Autodesk Inventor part; units mm, degrees
ref_plane "YZ Plane" through (0, 0, 0) normal (1, 0, 0) x (0, 1, 0)
ref_plane "XZ Plane" through (0, 0, 0) normal (0, 1, 0) x (-1, 0, 0)
ref_plane "XY Plane" through (0, 0, 0) normal (0, 0, 1) x (1, 0, 0)
sketch "Sketch1" plane through (0, 0, 0) normal (0, 0, 1) x (1, 0, 0)
  arc A0 (-44.1071, -48.8952) -> (-20.8929, -67.8977) centre (-32.5, -58.3964) ccw
  arc A1 (-43.869, -48.6061) -> (-44.1071, -48.8952) centre (0, -85) ccw
  line L0 (-36.9673, -34.403) -> (-43.869, -48.6061)
  arc A2 (-36.9673, -34.403) -> (-25, 17.6067) centre (-144, 17.6067) ccw
  line L1 (-25, 17.6067) -> (-25, 75)
  line L2 (-25, 75) -> (25, 75)
  line L3 (25, 75) -> (25, 17.6067)
  arc A3 (25, 17.6067) -> (36.9673, -34.403) centre (144, 17.6067) ccw
  line L4 (43.869, -48.6061) -> (36.9673, -34.403)
  arc A4 (44.1071, -48.8952) -> (43.869, -48.6061) centre (0, -85) ccw
  arc A5 (20.8929, -67.8977) -> (44.1071, -48.8952) centre (32.5, -58.3964) ccw
  arc A6 (20.8929, -67.8977) -> (-20.8929, -67.8977) centre (0, -85) ccw
  circle A7 centre (-16, 24) radius 2.1
  circle A8 centre (16, 60) radius 2.1
  circle A9 centre (-16, 60) radius 2.1
  circle A10 centre (16, 24) radius 2.1
  arc A11 (38.0714, -53.8358) -> (-38.0714, -53.8358) centre (0, -85) ccw
  arc A12 (-38.0714, -53.8358) -> (-26.9286, -62.957) centre (-32.5, -58.3964) ccw
  arc A13 (26.9286, -62.957) -> (-26.9286, -62.957) centre (0, -85) ccw
  arc A14 (26.9286, -62.957) -> (38.0714, -53.8358) centre (32.5, -58.3964) ccw
  circle A15 centre (0, -43) radius 7.1
  line L5 (0, -35.8) -> (0, -50.2) construction
  circle A16 centre (0, -85) radius 21.9
  line L6 (0, -63) -> (0, -213) construction
  line L7 (-42, -63) -> (-42, -213)
  line L8 (42, -213) -> (42, -63)
  arc A17 (42, -63) -> (-42, -63) centre (0, -63) ccw
  arc A18 (-42, -213) -> (42, -213) centre (0, -213) ccw
  point P0 (0, 0)
  point P1 (0, -138)
  dimension "d0" = 14.2
  dimension "d1" = 7.2
  dimension "d2" = 27
  dimension "d3" = 43.8
  dimension "d4" = 42
  dimension "d5" = 150
  dimension "d6" = 20
extrude "Extrusion1" add sketch "Sketch1" against normal blind 8 contours A15 | A16
sketch "Sketch2" plane through (0, -85, 0) normal (0, 0, 1) x (1, 0, 0)
  line L0 (-42, 22) -> (-42, -128)
  arc A0 (42, 22) -> (-42, 22) centre (0, 22) ccw
  line L1 (42, -128) -> (42, 22)
  arc A1 (-42, -128) -> (42, -128) centre (0, -128) ccw
  circle A2 centre (0, 0) radius 21.9
  circle A3 centre (0, 42) radius 7.1
  point P0 (0, 85)
extrude "Extrusion2" add sketch "Sketch2" along normal blind 10 contours A0 L1 A1 L0 | A2 | A3
sketch "Sketch4" plane through (0, -85, 0) normal (0, 0, -1) x (-1, 0, 0)
  circle A0 centre (0, 0) radius 21.9
  circle A1 centre (0, 42) radius 7.1
  arc A2 (-42, -128) -> (42, -128) centre (0, -128) ccw
  line L0 (42, 22) -> (42, -128)
  arc A3 (42, 22) -> (-42, 22) centre (0, 22) ccw
  line L1 (-42, -128) -> (-42, 22)
  arc A4 (-42, -128) -> (42, -128) centre (0, -128) ccw
  line L2 (42, -128) -> (-42, -128)
  line L3 (32, -128) -> (32, 12)
  arc A5 (42, 22) -> (-42, 22) centre (0, 22) ccw
  line L4 (32, 12) -> (42, 22)
  line L5 (0, -128) -> (0, 42) construction
  line L6 (-32, -128) -> (-32, 12)
  line L7 (-32, 12) -> (-42, 22)
  line L8 (22, -128) -> (22, -28)
  line L9 (22, -28) -> (32, -28)
  line L10 (-22, -128) -> (-22, -28)
  line L11 (-22, -28) -> (-32, -28)
  point P0 (0, 85)
  point P1 (-32, -28)
  dimension "d18" = 10
  dimension "d19" = 135
  dimension "d22" = 10
  dimension "d23" = 100
extrude "Extrusion3" cut sketch "Sketch4" against normal blind 10 contours L2 A2 | L1 L7 L6 L2 | L2 L3 L4 L0 | L6 L11 L10 L2 | L2 L8 L9 L3
sketch "Sketch5" plane through (0, -85, 10) normal (0, 0, 1) x (1, 0, 0)
  circle A0 centre (17, -73) radius 2.6
  circle A1 centre (17, -98) radius 2.6
  circle A2 centre (17, -123) radius 2.6
  point P0 (0, 85)
extrude "Extrusion4" cut sketch "Sketch5" against normal through all
ref_plane "Work Plane1" through (0, -85, 5) normal (0, 0, 1) x (1, 0, 0)
mirror "Mirror1" about plane through (0, -85, 5) normal (0, 0, 1) of "Extrusion1"
sketch "Sketch3" plane through (0, -43, -8) normal (0, 0, -1) x (-1, 0, 0)
  circle A0 centre (0, 0) radius 7.1
  point P0 (0, 43)
hole "Hole1" at (0, -43, -8) direction (0, 0, 1) diameter 8.2 end through all
properties part number "17_Khau_noi_tiep_cuoi" material "Stainless Steel, Austenitic"
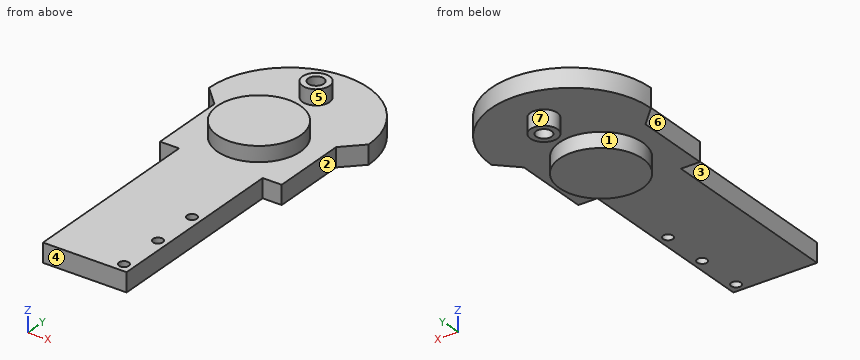
The listing builds one solid part. Answer for the finished solid, in the listing's coordinates (mm). Face numbers are marked on the shaded views. A direction names the side the tool comes from. Coordinates: 2 decimals unless noted, no trailing zeros. Write each loop counter-clockwise with the first axis right and the second up, starting at its lowest first coordinate (ties: lowest second). Pieces come first, ordered by that corner, then holes. Notation, with made-up numbers: M 33,38 L 86,38 A22 ccw 86,47 Z; hole C -35.5,74.25 d8. An arc over 180 degrees is marked long. Use a Markdown table: item, result. Add a question column.
1. Section A-A (x = 0) is taken. Give the vertices of the cut face in (y, z), plus the area to 3 significant figures.
2. Section C-C (y = -183) is taken. Give the vertices of the cut face in (x, z), plus the area to 3 significant figures.
3. Given P1, Ø11, axis at y = -157.5, z = 5.5, coming from the +X side; P2, Ø3, axis at y = -159, z = 6, coming from the -X side; P3, Ø1, axis at y = -79.5, z = 2.5, coming from the +X side, each flat-ended and moving along its own axis, determine where each tip first touches the part or whether it passes through.
4. Straight lines are drawn through the part: line 1 along X through (y, z) = (-158, 2.5); line 2 along Y through (x, z) = (0.5, -7); line 3 along Y through (x, z) = (17, 7.5). For each, find the intervals that lie inside material, in ascending order. Write a range as [from, to].
5. Section D-D (x = 17) is taken. Give the vertices of the cut face in (y, z).
6. For a pull along Y with two mould halves and no side action, classify the marked faces 4, 5, 6 and 7 as +Y half, -Y half, draft (parallel to the pull), parting line (faces both ways), or undercut.
7. Which of the six approach directions +Z, -Z, +X, -X, +Y, -Y give full straight-line access (tool end or side, diameter ignored) to the marked faces 1, 2 and 3?
8. Section B-B (z = -3) is taken. Give the vertices of the cut face in (x, y), plus the area to 3 significant figures.
Data:
| question | item | result |
|---|---|---|
| 1 | outline | M -213,0 L -106.9,0 L -106.9,-8 L -63.1,-8 L -63.1,0 L -50.1,0 L -50.1,-8 L -47.1,-8 L -47.1,18 L -50.1,18 L -50.1,10 L -63.1,10 L -63.1,18 L -106.9,18 L -106.9,10 L -213,10 Z; M -38.9,-8 L -35.9,-8 L -35.9,0 L -21,0 L -21,10 L -35.9,10 L -35.9,18 L -38.9,18 Z |
| 1 | area | 2,630 mm2 |
| 2 | outline | M -22,0 L 14.4,0 L 14.4,10 L -22,10 Z; M 19.6,0 L 22,0 L 22,10 L 19.6,10 Z |
| 2 | area | 388 mm2 |
| 3 | P1 | stops at x = 22 |
| 3 | P2 | stops at x = -22 |
| 3 | P3 | stops at x = 32 |
| 4 | line 1 | x = [-22, 14.4], [19.6, 22] |
| 4 | line 2 | y = [-106.89, -63.11], [-50.08, -47.07], [-38.93, -35.92] |
| 4 | line 3 | y = [-213, -210.6], [-205.4, -185.6], [-180.4, -160.6], [-155.4, -24.59] |
| 5 | outline | M -213,0 L -210.6,0 L -210.6,10 L -213,10 Z; M -205.4,0 L -185.6,0 L -185.6,10 L -205.4,10 Z; M -180.4,0 L -160.6,0 L -160.6,10 L -180.4,10 Z; M -155.4,0 L -98.81,0 L -98.81,-8 L -71.19,-8 L -71.19,0 L -24.59,0 L -24.59,10 L -71.19,10 L -71.19,18 L -98.81,18 L -98.81,10 L -155.4,10 Z |
| 6 | face 4 | -Y half |
| 6 | face 5 | undercut |
| 6 | face 6 | draft |
| 6 | face 7 | undercut |
| 7 | face 1 | -Z |
| 7 | face 2 | +Z, -Z, +X, -Y |
| 7 | face 3 | +Z, -Z, -X, -Y |
| 8 | outline | C 0,-85 d43.8; C 0,-43 d14.2; hole C 0,-43 d8.2 |
| 8 | area | 1,610 mm2 |
